```python
from build123d import *

# Parameters (mm, degrees)
F0_W     = 40.2
F0_H     = 20.4
F0_W_2   = 30.2
F0_H_2   = 10.4
F1_DEPTH = 30.9
F2_SIZE  = 2.5
F3_R     = 2
F4_R     = 0.5


with BuildPart() as f1:
    # F0 (on Top) → F1 (new body)
    with BuildSketch(Plane.XY):
        Rectangle(F0_W, F0_H)
        Rectangle(F0_W_2, F0_H_2, mode=Mode.SUBTRACT)
    extrude(amount=F1_DEPTH)

    # F2
    f2_edges = [f1.edges().sort_by_distance(p)[0] for p in [
        (-15.1, 0, 0),
        (0, -5.2, 0),
        (15.1, 0, 0),
        (0, 5.2, 0),
        (-15.1, 0, 30.9),
        (0, 5.2, 30.9),
        (15.1, 0, 30.9),
        (0, -5.2, 30.9),
    ]]
    chamfer(f2_edges, length=F2_SIZE)

    # F3
    f3_edges = [f1.edges().sort_by_distance(p)[0] for p in [
        (-20.1, -10.2, 15.45),
        (-20.1, 10.2, 15.45),
        (20.1, -10.2, 15.45),
        (20.1, 10.2, 15.45),
    ]]
    fillet(f3_edges, radius=F3_R)

    # F4
    f4_edges = [f1.edges().sort_by_distance(p)[0] for p in [
        (-15.1, 0, 28.4),
        (0, 5.2, 28.4),
        (15.1, 0, 28.4),
        (0, -5.2, 28.4),
        (0, 5.2, 2.5),
        (-15.1, 0, 2.5),
        (15.1, 0, 2.5),
        (0, -5.2, 2.5),
    ]]
    fillet(f4_edges, radius=F4_R)


solid = f1.part
```
Part model, mm, in its own coordinate system. A direction names the side the tool comes from. Give positions to 0.01 mm unless a question says otherwise; leave off trailing zeros. Order: outer loops, then holes, each group sorted by start corner. A loop starts at its lowest first (then second) coordinate and runs counter-clockwise, first axis right, second up. Notation, with made-up numbers: M 56.25,63 L 100.25,63 A31 cw 100.25,91 Z; hole C 53,-16 d2. An arc over 180 degrees is marked long. Use a Markdown table: item, result. Add a question column.
(1) Mould opens along Y. For faces 1 (the face through (0, -10.2, 15)), 2 (the face through (-2, -8, 30.9)), 3 (the face through (-15.1, 0, 15)) say: +Y half, -Y half, draft (parallel to the pull), parting line (faces both ways), or undercut.
(2) 3-axis set-ups, long thin cutter, end or side, ignore diameter. For faces 4 (the face through (-16.4, -0.1, 1.2)), 5 (the face through (-0.2, 6.5, 29.7)), 6 (the face through (15.1, 0, 15)): which of +Z, -Z, +X, -X, +Y, -Y reach the whole face in a straight line?
(3) Saw through at D-D, the plane x = 8. Give the cut face in (y, z).
(4) Drop flat-ended pins along their axis: P1, Ø4, axis at x = 3.5, y = 1.5, coming from the -Z side; P2, Ø1.5, axis at x = 5.5, y = 5, coming from the +Z side. Give the stop position or say it passes through.
(5) Probe line 1 along X through (y, z) = (-0.75, 12); line 2 along Y through (x, z) = (-13, 23); line 3 along X through (y, z) = (2.75, 29.5). List the from-to ranges inside material, lowest first. Write a range as [from, to].
(6) Saw through at B-B, the plane x = -16. Give the cut face in (y, z), and give its area (3 significant figures).
(7) Saw through at C-C, the plane z = 5. Give the cut face in (x, y).
(8) Saw through at A-A, the plane y = 0. Give the cut face in (x, z).
Answer key:
| question | item | result |
|---|---|---|
| 1 | face 1 | -Y half |
| 1 | face 2 | draft |
| 1 | face 3 | undercut |
| 2 | face 4 | -Z |
| 2 | face 5 | +Z |
| 2 | face 6 | +Z, -Z |
| 3 | outline | M -10.2,0 L -7.7,0 L -5.35,2.35 A0.5 ccw -5.2,2.71 L -5.2,28.19 A0.5 ccw -5.35,28.55 L -7.7,30.9 L -10.2,30.9 Z; M 5.2,2.71 A0.5 ccw 5.35,2.35 L 7.7,0 L 10.2,0 L 10.2,30.9 L 7.7,30.9 L 5.35,28.55 A0.5 ccw 5.2,28.19 Z |
| 4 | P1 | through |
| 4 | P2 | z = 28.95 |
| 5 | line 1 | [-20.1, -15.1], [15.1, 20.1] |
| 5 | line 2 | [-10.2, -5.2], [5.2, 10.2] |
| 5 | line 3 | [-20.1, -16.2], [16.2, 20.1] |
| 6 | outline | M -10.2,0 L -7.7,0 L -6.1,1.6 L 6.1,1.6 L 7.7,0 L 10.2,0 L 10.2,30.9 L 7.7,30.9 L 6.1,29.3 L -6.1,29.3 L -7.7,30.9 L -10.2,30.9 Z |
| 6 | area | 586 mm^2 |
| 7 | outline | M -20.1,-8.2 A2 ccw -18.1,-10.2 L 18.1,-10.2 A2 ccw 20.1,-8.2 L 20.1,8.2 A2 ccw 18.1,10.2 L -18.1,10.2 A2 ccw -20.1,8.2 Z; hole M -15.1,-5.2 L 15.1,-5.2 L 15.1,5.2 L -15.1,5.2 Z |
| 8 | outline | M -20.1,0 L -17.6,0 L -15.25,2.35 A0.5 ccw -15.1,2.71 L -15.1,28.19 A0.5 ccw -15.25,28.55 L -17.6,30.9 L -20.1,30.9 Z; M 15.1,2.71 A0.5 ccw 15.25,2.35 L 17.6,0 L 20.1,0 L 20.1,30.9 L 17.6,30.9 L 15.25,28.55 A0.5 ccw 15.1,28.19 Z |
